Verification items for the finished model (mm, model axes). Give positions to 0.01 mm unless a question says otherwise; leave off trailing zeros. Loops run counter-clockwise (first coordinate to the right, second up) from the corner with the lowest first, then second, coordinate; pieces in that order, holes last. Notation, with made-up numbers: M 64,45.25 L 72,45.25 A6 cw 72,52.25 Z; hole C 44.25,5.5 d5. An arc over 180 degrees is marked long. Use a Markdown table: item, result.
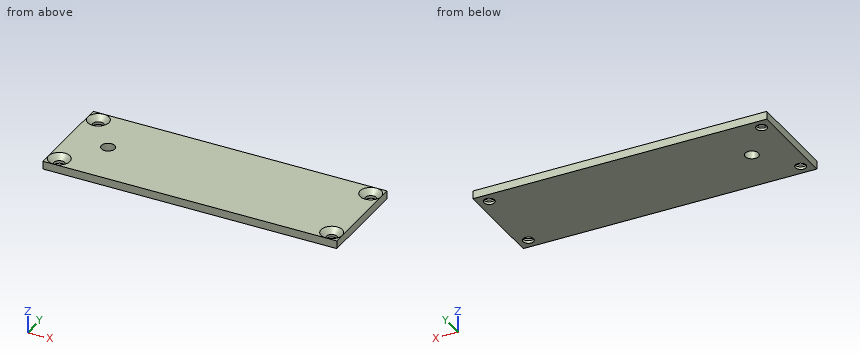
from build123d import *

# Parameters (mm, degrees)
SKETCH_W        = 110
SKETCH_H        = 36
PAD_DEPTH       = 3
SKETCH002_R     = 2
POCKET_DEPTH    = 3
CHAMFER_SIZE    = 1.99
SKETCH003_R     = 2.5
POCKET001_DEPTH = 3


with BuildPart() as part:
    # Sketch → Pad (new body)
    with BuildSketch(Plane.XY):
        Rectangle(SKETCH_W, SKETCH_H)
    extrude(amount=PAD_DEPTH)

    # Sketch002 (on Face6 of Pad) → Pocket (cut)
    with BuildSketch(Plane.XY.offset(3)):
        with Locations((-51, 14)):
            Circle(SKETCH002_R)
        with Locations((-51, -14)):
            Circle(SKETCH002_R)
        with Locations((51, -14)):
            Circle(SKETCH002_R)
        with Locations((51, 14)):
            Circle(SKETCH002_R)
    extrude(amount=-POCKET_DEPTH, mode=Mode.SUBTRACT)

    # Chamfer
    chamfer_edges = [part.edges().sort_by_distance(p)[0] for p in [
        (-53, 14, 3),
        (-53, -14, 3),
        (49, -14, 3),
        (49, 14, 3),
    ]]
    chamfer(chamfer_edges, length=CHAMFER_SIZE)

    # Sketch003 (on Face1 of Chamfer) → Pocket001 (cut)
    with BuildSketch(Plane.XY.offset(3)):
        with Locations((-40, 0)):
            Circle(SKETCH003_R)
    extrude(amount=-POCKET001_DEPTH, mode=Mode.SUBTRACT)


solid = part.part
(1) Cross-section at C-C on x = -40. Record the cut outline in (y, z).
Results below:
| item | result |
|---|---|
| outline | M -18,0 L -2.5,0 L -2.5,3 L -18,3 Z; M 2.5,0 L 18,0 L 18,3 L 2.5,3 Z |
(2) Gauge pin test, flat end, axial feed: P1, Ø4.5, axis at x = 51, y = -14, coming from the -Z side. Record the tip position at first contact, or that the pin passes through.
Results below:
| item | result |
|---|---|
| P1 | z = 0 |
(3) Cross-section at A-A on y = -14. State how many separate pieces and enclosed holes the cut face has, then the cut area to 3 significant figures.
Results below:
| item | result |
|---|---|
| separate pieces | 3 |
| enclosed holes | 0 |
| area | 298 mm^2 |
(4) Material ranges on line 1 (Y direction, x = -51, z = 0.5); line 2 (X direction, y = 12.5, z = 1.15); line 3 (Y direction, x = -42, z = 1.5), recorded low to high.
Results below:
| item | result |
|---|---|
| line 1 | -18 to -16, -12 to 12, 16 to 18 |
| line 2 | -55 to -52.53, -49.47 to 49.47, 52.53 to 55 |
| line 3 | -18 to -1.5, 1.5 to 18 |
